Part print with two shaded views. Sizes in mm from the minimum x, y, z corner. A direction names the side the tool comes from. Round coordinates to 2 decimals unless told otherwise and drop trailing zeros. Loops run counter-clockwise (first coordinate to the right, second up) from the corner with the lowest first, then second, coordinate; pieces in that order, holes last. Notation, with made-up numbers: (49, 11) -> (62, 11) arc R8 ccw to (62, 24) -> close; hole circle Ø7 at (14, 37.5). An arc over 180 degrees is marked (long way). Use a Markdown table: item, result. Add a question column.
Item 1: Cut at C-C, the plane x = 2. List the corners of the cut face in (y, z), plus the area to 3 significant figures.
Item 2: Cut at D-D, the plane y = 11.25. List the corners of the cut face in (x, z).
Item 3: Flat gauge pins, fed straight in: pin 1 (3 mm diameter, centred on x = 3, z = 4.5, fed in from -Y); pin 2 (3 mm diameter, centred on x = 6, z = 2, fed in from +Y); pin 3 (1.5 mm diameter, centred on x = 3.5, y = 2, fed in from +Z). Where does each tip first touch, or does it go through?
Item 4: Two-plate mould, pull along Z, no slides. Class the marked faces 1, 2 and 3: pulls with the +Z half, pulls with the -Z half, needs draft (parallel to the pull), parting line crosses it, or undercut.
Item 5: Which spindle directions (+Z, -Z, +X, -X, +Y, -Y) get a long thin tool onto all of the face, cutting with end or side? Do the marked faces 4, 5 and 6. Say none if no direction does.
Item 6: Probe line 1 (Z direction, x = 0.7, y = 7.5); line 2 (Z direction, x = 5.4, y = 7.5); line 3 (Y direction, x = 1.75, z = 6.5). List the from-to ranges inside material, lowest first. Write a range as [from, to].
Item 7: Cut at A-A, the plane y = 7.5. List the corners of the cut face in (x, z).
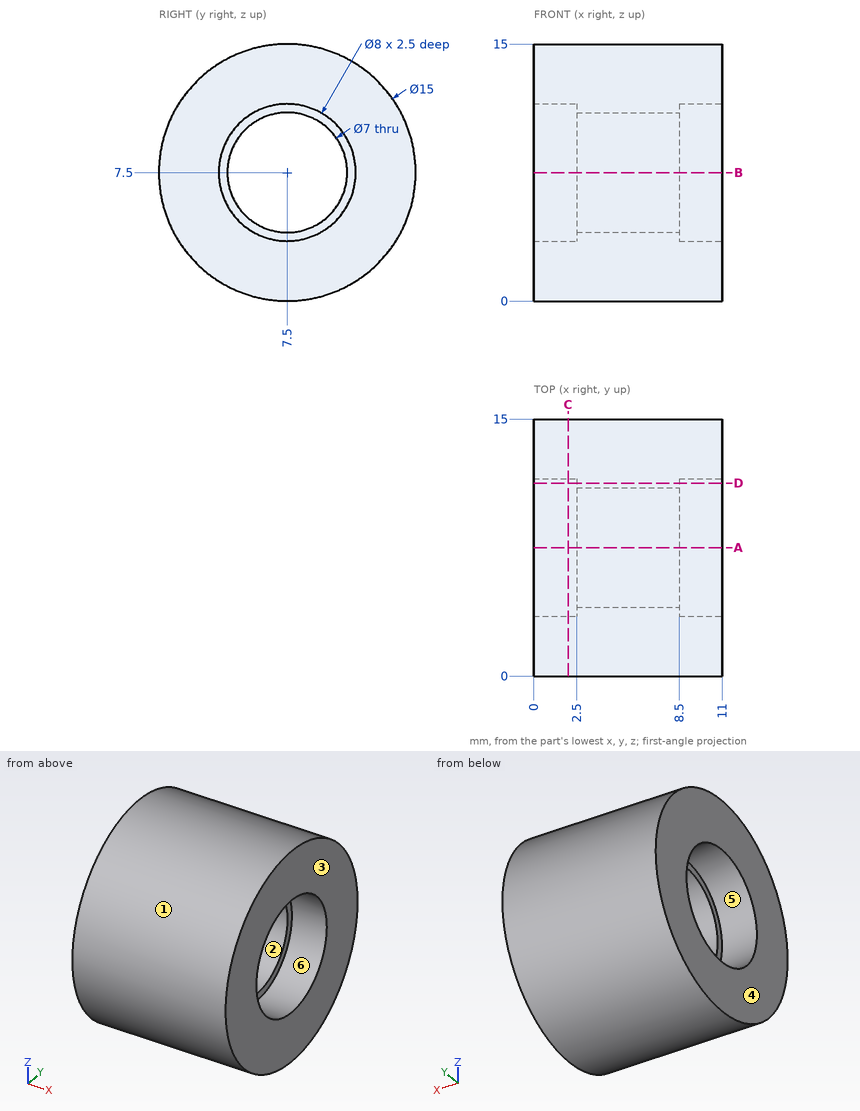
A:
| question | item | result |
|---|---|---|
| 1 | outline | circle Ø15 at (7.5, 7.5); hole circle Ø8 at (7.5, 7.5) |
| 1 | area | 126 mm^2 |
| 2 | outline | (0, 1) -> (11, 1) -> (11, 6.11) -> (8.5, 6.11) -> (8.5, 8.89) -> (11, 8.89) -> (11, 14) -> (0, 14) -> (0, 8.89) -> (2.5, 8.89) -> (2.5, 6.11) -> (0, 6.11) -> close |
| 3 | pin 1 | stops at y = 0.15 |
| 3 | pin 2 | stops at y = 13.84 |
| 3 | pin 3 | stops at z = 13.3 |
| 4 | face 1 | parting line crosses it |
| 4 | face 2 | undercut |
| 4 | face 3 | needs draft |
| 5 | face 4 | +Z, -Z, -X, +Y, -Y |
| 5 | face 5 | -X |
| 5 | face 6 | +X |
| 6 | line 1 | z = [0, 3.5], [11.5, 15] |
| 6 | line 2 | z = [0, 4], [11, 15] |
| 6 | line 3 | y = [0.07, 3.63], [11.37, 14.93] |
| 7 | outline | (0, 0) -> (11, 0) -> (11, 3.5) -> (8.5, 3.5) -> (8.5, 4) -> (2.5, 4) -> (2.5, 3.5) -> (0, 3.5) -> close; (0, 11.5) -> (2.5, 11.5) -> (2.5, 11) -> (8.5, 11) -> (8.5, 11.5) -> (11, 11.5) -> (11, 15) -> (0, 15) -> close |
